Input: part model. Units: mm. Frame: model coordinates. Face numbers are marked on the shaded views. A direction names the side the tool comes from. Coordinates: 2 decimals unless noted, no trailing zeros. Write each loop counter-clockwise with the first axis right and the second up, starting at its lowest first coordinate (ties: lowest second). Pieces come first, ordered by that corner, then holes. Notation, with made-up numbers: (89.25, 74.25) - (125.25, 74.25) arc R18 cw to (125.25, 94.25) - close; hole circle Ø3 at (82.25, 81.5). An arc over 180 degrees is marked (long way). Put each result on its own line as item: value. Start each with the question number.
1. Cut plane B-B, the plane z = 18.25. Return loops of the section in (x, y).
2. Cut plane D-D, the plane y = -1. Return loops of the section in (x, z), and give its area (3 significant figures).
3. Pin query (flat end, axial travel): pin 1 (3 mm diameter, centred on x = 0.5, z = 21, fed in from +Y); pin 2 (2.5 mm diameter, centred on x = -1, y = -1.5, fed in from +Z); pin 3 (3 mm diameter, centred on x = 0, y = 0, fed in from +Z); pin 4 (3 mm diameter, centred on y = -1.5, z = 25, fed in from -X). Return the tip coordinate at first contact, or that it passes through.
4. Line query: line 1 (Y direction, x = 0, z = 14.75); line 2 (Y direction, x = 10, z = 27); line 3 (Z direction, x = 4, y = -3.25). Output: solid intervals per line, ascending.
5. Access query for the marked faces 4, 5, 6 and 7. Directions: +Z, -Z, +X, -X, +Y, -Y. A direction counts if a zero-diameter tool reaches every point of the face in a straight line with its end or side. Return the directions, or none.
6. Pull-direction query (Y, two-part tool) for the marked faces 1, 2 and 3; classes: released by +Y, released by -Y, zero draft, split by the parting line, or undercut.
7. Cut plane A-A, the plane y = 0.5. Return loops of the section in (x, z).
8. Cut plane C-C, the plane z = 25. Return loops of the section in (x, y).
from build123d import *

# Parameters (mm, degrees)
EXTRUDE_1_DEPTH     = 30
SKETCH_2_W          = 9
SKETCH_2_H          = 8.937793365
SKETCH_2_H_2        = 10.067856953
CUT_EXTRUDE_1_DEPTH = 15
SKETCH_3_R          = 2
CUT_EXTRUDE_2_DEPTH = 32


with BuildPart() as part:
    # 草图1 → 凸台-拉伸1 (new body)
    with BuildSketch(Plane.XY):
        with BuildLine():
            Line((4, 0), (20, 0))
            Line((20, 0), (20, -4))
            Line((20, -4), (0, -4))
            ThreePointArc((0, -4), (-2.828427125, 2.828427125), (4, 0))
        make_face()
    extrude(amount=EXTRUDE_1_DEPTH)

    # 草图2 → 切除-拉伸1 (cut)
    with BuildSketch(Plane.XZ.offset(4)):
        with Locations((0, 26.468896683)):
            Rectangle(SKETCH_2_W, SKETCH_2_H)
        with Locations((0, 2.966071524)):
            Rectangle(SKETCH_2_W, SKETCH_2_H_2)
    extrude(amount=-CUT_EXTRUDE_1_DEPTH, mode=Mode.SUBTRACT)

    # 草图3 → 切除-拉伸2 (cut)
    with BuildSketch(Plane(origin=(0, 0, 0), x_dir=(-1, 0, 0), z_dir=(0, 0, -1))):
        Circle(SKETCH_3_R)
    extrude(amount=-CUT_EXTRUDE_2_DEPTH, mode=Mode.SUBTRACT)


solid = part.part
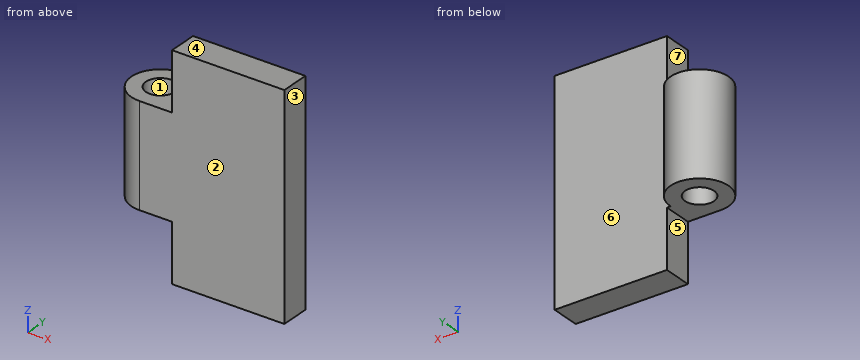
Report:
1. outline: (0, -4) - (20, -4) - (20, 0) - (4, 0) arc R4 ccw (long way) to start; hole circle Ø4 at (0, 0)
2. outline: (-3.87, 8) - (-1.73, 8) - (-1.73, 22) - (-3.87, 22) - close; (1.73, 8) - (4.5, 8) - (4.5, 0) - (20, 0) - (20, 30) - (4.5, 30) - (4.5, 22) - (1.73, 22) - close
2. area: 534 mm^2
3. pin 1: stops at y = 4
3. pin 2: stops at z = 22
3. pin 3: passes through
3. pin 4: stops at x = 4.5
4. line 1: y = -4 to -2, 2 to 4
4. line 2: y = -4 to 0
4. line 3: z = 8 to 22
5. face 4: +Z, +X, -X, +Y, -Y
5. face 5: -Z, -X, +Y, -Y
5. face 6: +Z, -Z, +X, +Y
5. face 7: +Z, -X, +Y, -Y
6. face 1: undercut
6. face 2: released by -Y
6. face 3: zero draft
7. outline: (-3.97, 8) - (-1.94, 8) - (-1.94, 22) - (-3.97, 22) - close; (1.94, 8) - (3.97, 8) - (3.97, 22) - (1.94, 22) - close
8. outline: (4.5, -4) - (20, -4) - (20, 0) - (4.5, 0) - close
